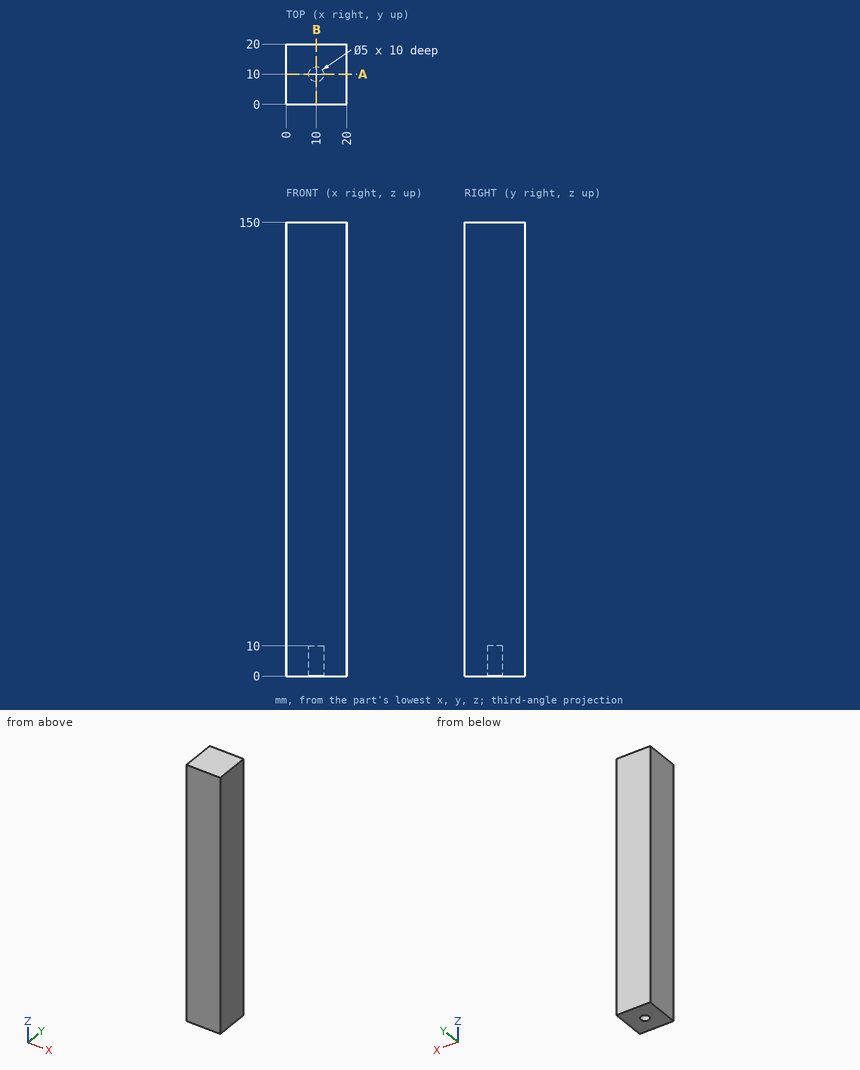
Check sheet for the drawn part. Datum: minimum x, y, z corner. Units: mm. Round coordinates to 2 decimals unless told otherwise and drop trailing zeros. Loops run counter-clockwise (first coordinate to the right, second up) from the corner with the lowest first, then second, coordinate; pieces in that order, holes last. Notation, with made-up numbers: (88.5, 48) -> (129.5, 48) arc R6 ccw to (129.5, 55) -> close; hole circle Ø9 at (64.25, 49.5). An arc over 180 degrees is marked (long way). Put each result on its own line as item: value. Start each with the question number.
1. Gauge pin test, flat end, axial feed: pin 1 (2.5 mm diameter, centred on x = 10, y = 11, fed in from -Z). Record the tip position at first contact, or that the pin passes through.
2. Scan lines: probe 1 along Y at (x, z) = (10, 7.5); probe 2 along Z at (x, y) = (12.25, 9.25). Record each from-to range of solid material in increasing order.
3. Section check A-A (y = 10). Enter the section's corners in (x, z).
Findings:
1. pin 1: stops at z = 10
2. probe 1: y = 0 to 7.5, 12.5 to 20
2. probe 2: z = 10 to 150
3. outline: (0, 0) -> (7.5, 0) -> (7.5, 10) -> (12.5, 10) -> (12.5, 0) -> (20, 0) -> (20, 150) -> (0, 150) -> close
